The figure shows three views and two pictorial views of one solid part (mm, origin at its lowest corner). Answer the questions. Coordinates: 2 decimals unless noted, no trailing zeros. Loops run counter-clockwise (first coordinate to the right, second up) from the corner with the lowest first, then second, coordinate; pieces in that order, holes last. Notation, with made-up numbers: M 3,-37.75 L 36,-37.75 A15 cw 36,-8.75 Z; hole C 65.5,30.5 d2. An arc over 180 degrees is marked long. Return JSON: item names as keys, results as strings. Group by question number.
1. Given P1, Ø4, axis at x = 155.5, y = 20.5, coming from the +Z side; P2, Ø5, axis at x = 179.5, y = 11, coming from the +Z side; P3, Ø3, axis at x = 169.5, y = 44, coming from the -Z side, each flat-ended and moving along its own axis, determine where each tip first touches the part or whether it passes through.
2. The mould has two halves that part along X. Classify the marked faces 1, 2, 3 and 4: pulls with the +X half, pulls with the -X half, needs draft (parallel to the pull), parting line crosses it, or undercut.
3. Straight lines are drawn through the part: L1, parallel to X at y = 73, z = 44; L2, parallel to Z at x = 110.5, y = 48; L3, parallel to Y at x = 59.5, z = 23. For each, find the intervals that lie inside material, in ascending order. Write a range as from..to.
4. Section A-A (y = 6) is taken. Write down the section's boundary in (x, z).
5. Section B-B (z = 75) is taken. Write down the section's boundary in (x, y).
6. Section C-C (y = 40) is taken. Write down the section's boundary in (x, z), then the cut area to 3 significant figures.
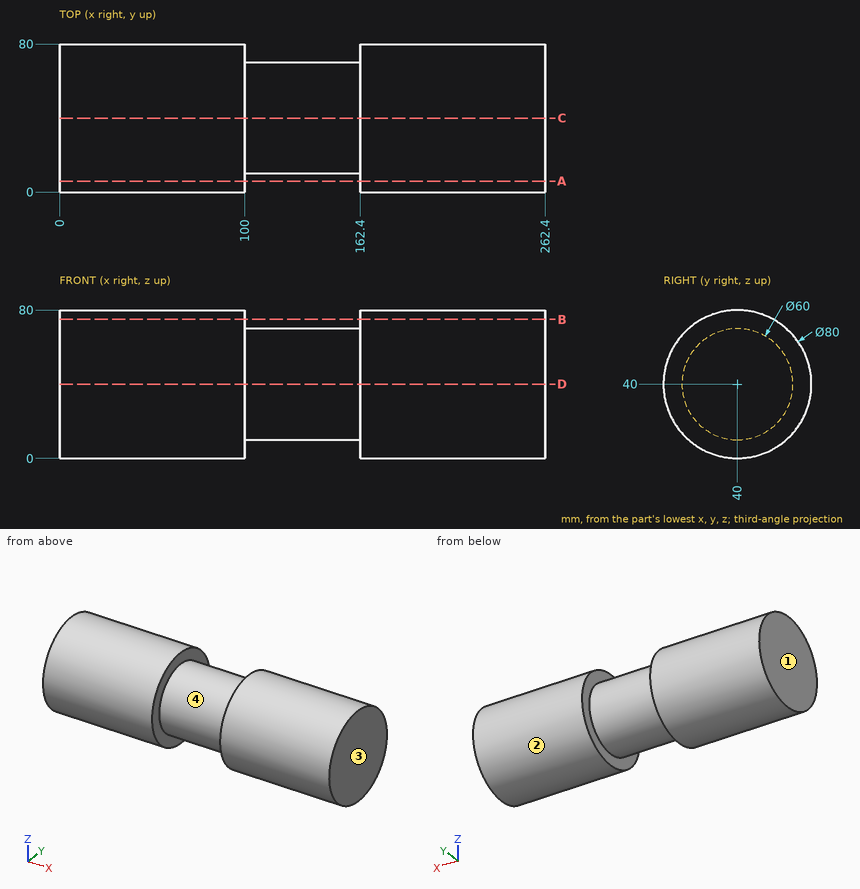
Worked out:
{
 "1": {"P1": "z = 64.37", "P2": "z = 69.96", "P3": "z = 0.08"},
 "2": {"face 1": "pulls with the -X half", "face 2": "needs draft", "face 3": "pulls with the +X half", "face 4": "undercut"},
 "3": {"L1": "0..100, 162.4..262.4", "L2": "11.09..68.91", "L3": "3.79..76.21"},
 "4": {"outline": "M 0,18.93 L 100,18.93 L 100,61.07 L 0,61.07 Z; M 162.4,18.93 L 262.4,18.93 L 262.4,61.07 L 162.4,61.07 Z"},
 "5": {"outline": "M 0,20.64 L 100,20.64 L 100,59.36 L 0,59.36 Z; M 162.4,20.64 L 262.4,20.64 L 262.4,59.36 L 162.4,59.36 Z"},
 "6": {"outline": "M 0,0 L 100,0 L 100,10 L 162.4,10 L 162.4,0 L 262.4,0 L 262.4,80 L 162.4,80 L 162.4,70 L 100,70 L 100,80 L 0,80 Z", "area": "19,700 mm^2"}
}
